Geometry check sheet. Reference: the model listing, model coordinates, mm. Give positions to 0.01 mm unless a question says otherwise; leave off trailing zeros. Loops run counter-clockwise (first coordinate to the right, second up) from the corner with the lowest first, then second, coordinate; pieces in that order, holes last. Notation, with made-up numbers: (11.25, 65) - (63.25, 65) arc R12 cw to (63.25, 79) - close; hole circle Ø6 at (82.25, -22.75). An arc over 180 degrees is marked (long way). Use a Markdown table: item, result. Add a question column.
1. Cross-section at C-C on y = 12. Enter the section's corners in (x, z), and give its area (3 significant figures).
2. Material ranges on L1, parallel to Z at x = -0.25, y = 14; L2, parallel to X at y = 7, z = 7.5; L3, parallel to Z at x = 9.5, y = 37, recorded low to high.
3. Depth check by flat-ended pin: P1, Ø5, axis at x = -11, y = 23.5, coming from the +Z side; P2, Ø8, axis at x = 1, y = 70, coming from the +Z side; P3, Ø1.5, axis at x = -7.5, y = 30.5, coming from the -Z side. Enter the tip coordinate at first touch or a pass-through.
4. Cross-section at B-B on y = 61.5. Enter the section's corners in (x, z), and give its area (3 significant figures).
5. Cross-section at A-A on x = 0. Enter the section's corners in (y, z), and give its area (3 significant figures).
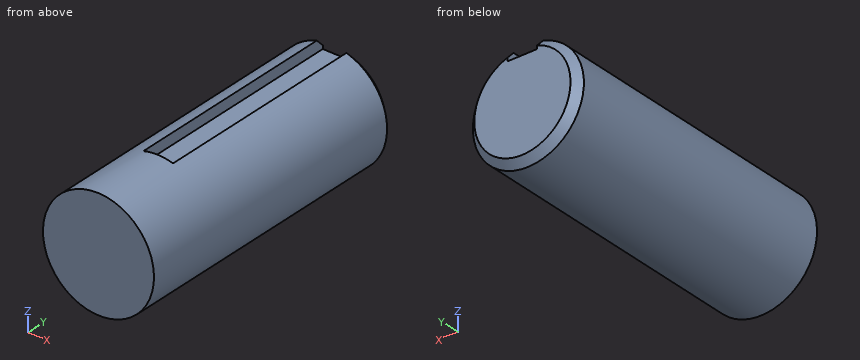
from build123d import *

# Parameters (mm, degrees)
SKETCH1_R           = 15
BOSS_EXTRUDE1_DEPTH = 80
CHAMFER1_SIZE       = 2
CUT_EXTRUDE1_START  = -60
CUT_EXTRUDE1_DEPTH  = 60


with BuildPart() as part:
    # Sketch1 → Boss-Extrude1 (new body)
    with BuildSketch(Plane(origin=(0, 0, 0), x_dir=(-1, 0, 0), z_dir=(0, 1, 0))):
        with Locations(Location((0, 0, 0), (0, 0, 90))):
            Circle(SKETCH1_R)
    extrude(amount=BOSS_EXTRUDE1_DEPTH)

    # Chamfer1
    chamfer1_edges = [part.edges().sort_by_distance(p)[0] for p in [
        (0, 80, -15),
    ]]
    chamfer(chamfer1_edges, length=CHAMFER1_SIZE)

    # Sketch3 → Cut-Extrude1 (cut)
    with BuildSketch(Plane(origin=(0, 80, 0), x_dir=(-1, 0, 0), z_dir=(0, 1, 0)).offset(CUT_EXTRUDE1_START)):
        with BuildLine():
            Line((-4, 14.456832295), (-4, 11.456832295))
            Line((-4, 11.456832295), (4, 11.456832295))
            Line((4, 11.456832295), (4, 14.456832295))
            ThreePointArc((4, 14.456832295), (0, 15), (-4, 14.456832295))
        make_face()
    extrude(amount=CUT_EXTRUDE1_DEPTH, mode=Mode.SUBTRACT)


solid = part.part
Values found:
| question | item | result |
|---|---|---|
| 1 | outline | circle Ø30 at (0, 0) |
| 1 | area | 707 mm2 |
| 2 | L1 | z = -15 to 15 |
| 2 | L2 | x = -12.99 to 12.99 |
| 2 | L3 | z = -11.61 to 11.61 |
| 3 | P1 | stops at z = 12.36 |
| 3 | P2 | stops at z = 14.46 |
| 3 | P3 | stops at z = -13.4 |
| 4 | outline | (-4, 11.46) - (-4, 14.46) arc R15 ccw (long way) to (4, 14.46) - (4, 11.46) - close |
| 4 | area | 680 mm2 |
| 5 | outline | (0, -15) - (78, -15) - (80, -13) - (80, 11.46) - (20, 11.46) - (20, 15) - (0, 15) - close |
| 5 | area | 2,190 mm2 |
